Read the model definition and answer for the solid it produces. Units are mm, in the model's axes. Face numbers are marked on the shaded views. A direction names the side the tool comes from. Give positions to 0.01 mm unless a question says otherwise; leave off trailing zeros. Write each loop counter-clockwise with the first axis right and the second up, starting at its lowest first coordinate (ties: lowest second). Pieces come first, ordered by that corner, then holes. Notation, with made-up numbers: M 33,73 L 60,73 A16 ccw 60,77 Z; hole C 36.25,-25.75 d10. An arc over 180 degrees is marked long. Use a Markdown table: item, result. Add a question column.
Item 1: A cutting plane is placed at B-B on x = -33. Count the separate pieces of the cut face and the enclosed holes in it, then the cut area to 3 significant figures.
Item 2: A cutting plane is placed at A-A on z = 4.25. Determine the outline of the cut face in (x, y).
Item 3: Given P1, Ø13, axis at x = 0.01, y = -11.72, coming from the -Z side; P2, Ø4, axis at x = 51, y = 19.5, coming from the +Z side, each flat-ended and moving along its own axis, determine where each tip first touches the part or whether it passes through.
Item 4: A cutting plane is placed at C-C on x = -70. Determine the outline of the cut face in (y, z), then the cut area to 3 significant figures.
Item 5: For the marked faces 1 and 2, determine the directions among +Z, -Z, +X, -X, +Y, -Y from which every point of the face is accessible in a straight line to the end or side of a thin tool.
Item 6: Consider probe 1 along Y at (x, z) = (-70, 1.2); probe 2 along Y at (x, z) = (47, 5.75); probe 3 along Z at (x, y) = (-17, 66). Determine where each line is inside the solid, lowest interval first. Write a range as [from, to].
Item 7: A cutting plane is placed at D-D on y = 62.5. Determine the outline of the cut face in (x, z).
from build123d import *

# Parameters (mm, degrees)
SKETCH_W      = 150
SKETCH_H      = 150
SKETCH_R      = 4
SKETCH_R_2    = 2
PAD_DEPTH     = 3
SKETCH001_R   = 4
SKETCH001_R_2 = 2
PAD001_DEPTH  = 4


with BuildPart() as part:
    # Sketch → Pad (new body)
    with BuildSketch(Plane.XY):
        Rectangle(SKETCH_W, SKETCH_H)
        with Locations((-23.457463, 46.865997)):
            Circle(SKETCH_R, mode=Mode.SUBTRACT)
        with Locations((-11.738286, 46.871353)):
            Circle(SKETCH_R, mode=Mode.SUBTRACT)
        with Locations((-0.019109, 46.876709)):
            Circle(SKETCH_R, mode=Mode.SUBTRACT)
        with Locations((11.700068, 46.882065)):
            Circle(SKETCH_R, mode=Mode.SUBTRACT)
        with Locations((23.419245, 46.887421)):
            Circle(SKETCH_R, mode=Mode.SUBTRACT)
        with Locations((-35.173599, 35.141463)):
            Circle(SKETCH_R, mode=Mode.SUBTRACT)
        with Locations((-23.454422, 35.146819)):
            Circle(SKETCH_R, mode=Mode.SUBTRACT)
        with Locations((-11.735245, 35.152175)):
            Circle(SKETCH_R, mode=Mode.SUBTRACT)
        with Locations((-0.016068, 35.157531)):
            Circle(SKETCH_R, mode=Mode.SUBTRACT)
        with Locations((11.703109, 35.162887)):
            Circle(SKETCH_R, mode=Mode.SUBTRACT)
        with Locations((23.422286, 35.168243)):
            Circle(SKETCH_R, mode=Mode.SUBTRACT)
        with Locations((35.141463, 35.173599)):
            Circle(SKETCH_R, mode=Mode.SUBTRACT)
        with Locations((-46.88742, 23.41693)):
            Circle(SKETCH_R, mode=Mode.SUBTRACT)
        with Locations((-35.168243, 23.422286)):
            Circle(SKETCH_R, mode=Mode.SUBTRACT)
        with Locations((-23.449066, 23.427642)):
            Circle(SKETCH_R, mode=Mode.SUBTRACT)
        with Locations((-11.729889, 23.432998)):
            Circle(SKETCH_R, mode=Mode.SUBTRACT)
        with Locations((-0.010712, 23.438354)):
            Circle(SKETCH_R, mode=Mode.SUBTRACT)
        with Locations((11.708465, 23.44371)):
            Circle(SKETCH_R, mode=Mode.SUBTRACT)
        with Locations((23.427642, 23.449066)):
            Circle(SKETCH_R, mode=Mode.SUBTRACT)
        with Locations((35.146819, 23.454422)):
            Circle(SKETCH_R, mode=Mode.SUBTRACT)
        with Locations((46.865996, 23.459778)):
            Circle(SKETCH_R, mode=Mode.SUBTRACT)
        with Locations((-46.882064, 11.697753)):
            Circle(SKETCH_R, mode=Mode.SUBTRACT)
        with Locations((-35.162887, 11.703109)):
            Circle(SKETCH_R, mode=Mode.SUBTRACT)
        with Locations((-23.44371, 11.708465)):
            Circle(SKETCH_R, mode=Mode.SUBTRACT)
        with Locations((-11.724533, 11.713821)):
            Circle(SKETCH_R, mode=Mode.SUBTRACT)
        with Locations((-0.005356, 11.719177)):
            Circle(SKETCH_R, mode=Mode.SUBTRACT)
        with Locations((11.713821, 11.724533)):
            Circle(SKETCH_R, mode=Mode.SUBTRACT)
        with Locations((23.432998, 11.729889)):
            Circle(SKETCH_R, mode=Mode.SUBTRACT)
        with Locations((35.152175, 11.735245)):
            Circle(SKETCH_R, mode=Mode.SUBTRACT)
        with Locations((46.871352, 11.740601)):
            Circle(SKETCH_R, mode=Mode.SUBTRACT)
        with Locations((-46.876708, -0.021424)):
            Circle(SKETCH_R, mode=Mode.SUBTRACT)
        with Locations((-35.157531, -0.016068)):
            Circle(SKETCH_R, mode=Mode.SUBTRACT)
        with Locations((-23.438354, -0.010712)):
            Circle(SKETCH_R, mode=Mode.SUBTRACT)
        with Locations((-11.719177, -0.005356)):
            Circle(SKETCH_R, mode=Mode.SUBTRACT)
        Circle(SKETCH_R, mode=Mode.SUBTRACT)
        with Locations((11.719177, 0.005356)):
            Circle(SKETCH_R, mode=Mode.SUBTRACT)
        with Locations((23.438354, 0.010712)):
            Circle(SKETCH_R, mode=Mode.SUBTRACT)
        with Locations((35.157531, 0.016068)):
            Circle(SKETCH_R, mode=Mode.SUBTRACT)
        with Locations((46.876708, 0.021424)):
            Circle(SKETCH_R, mode=Mode.SUBTRACT)
        with Locations((-46.871352, -11.740601)):
            Circle(SKETCH_R, mode=Mode.SUBTRACT)
        with Locations((-35.152175, -11.735245)):
            Circle(SKETCH_R, mode=Mode.SUBTRACT)
        with Locations((-23.432998, -11.729889)):
            Circle(SKETCH_R, mode=Mode.SUBTRACT)
        with Locations((-11.713821, -11.724533)):
            Circle(SKETCH_R, mode=Mode.SUBTRACT)
        with Locations((0.005356, -11.719177)):
            Circle(SKETCH_R, mode=Mode.SUBTRACT)
        with Locations((11.724533, -11.713821)):
            Circle(SKETCH_R, mode=Mode.SUBTRACT)
        with Locations((23.44371, -11.708465)):
            Circle(SKETCH_R, mode=Mode.SUBTRACT)
        with Locations((35.162887, -11.703109)):
            Circle(SKETCH_R, mode=Mode.SUBTRACT)
        with Locations((46.882064, -11.697753)):
            Circle(SKETCH_R, mode=Mode.SUBTRACT)
        with Locations((-46.865996, -23.459778)):
            Circle(SKETCH_R, mode=Mode.SUBTRACT)
        with Locations((-35.146819, -23.454422)):
            Circle(SKETCH_R, mode=Mode.SUBTRACT)
        with Locations((-23.427642, -23.449066)):
            Circle(SKETCH_R, mode=Mode.SUBTRACT)
        with Locations((-11.708465, -23.44371)):
            Circle(SKETCH_R, mode=Mode.SUBTRACT)
        with Locations((0.010712, -23.438354)):
            Circle(SKETCH_R, mode=Mode.SUBTRACT)
        with Locations((11.729889, -23.432998)):
            Circle(SKETCH_R, mode=Mode.SUBTRACT)
        with Locations((23.449066, -23.427642)):
            Circle(SKETCH_R, mode=Mode.SUBTRACT)
        with Locations((35.168243, -23.422286)):
            Circle(SKETCH_R, mode=Mode.SUBTRACT)
        with Locations((46.88742, -23.41693)):
            Circle(SKETCH_R, mode=Mode.SUBTRACT)
        with Locations((-35.141463, -35.173599)):
            Circle(SKETCH_R, mode=Mode.SUBTRACT)
        with Locations((-23.422286, -35.168243)):
            Circle(SKETCH_R, mode=Mode.SUBTRACT)
        with Locations((-11.703109, -35.162887)):
            Circle(SKETCH_R, mode=Mode.SUBTRACT)
        with Locations((0.016068, -35.157531)):
            Circle(SKETCH_R, mode=Mode.SUBTRACT)
        with Locations((11.735245, -35.152175)):
            Circle(SKETCH_R, mode=Mode.SUBTRACT)
        with Locations((23.454422, -35.146819)):
            Circle(SKETCH_R, mode=Mode.SUBTRACT)
        with Locations((35.173599, -35.141463)):
            Circle(SKETCH_R, mode=Mode.SUBTRACT)
        with Locations((-23.416872, -46.88742)):
            Circle(SKETCH_R, mode=Mode.SUBTRACT)
        with Locations((-11.697695, -46.882064)):
            Circle(SKETCH_R, mode=Mode.SUBTRACT)
        with Locations((0.021482, -46.876708)):
            Circle(SKETCH_R, mode=Mode.SUBTRACT)
        with Locations((11.740659, -46.871352)):
            Circle(SKETCH_R, mode=Mode.SUBTRACT)
        with Locations((23.459836, -46.865996)):
            Circle(SKETCH_R, mode=Mode.SUBTRACT)
        with Locations((-47.999982, 47.941119)):
            Circle(SKETCH_R_2, mode=Mode.SUBTRACT)
        with Locations((48, 48)):
            Circle(SKETCH_R_2, mode=Mode.SUBTRACT)
        with Locations((-47.941101, -48.058863)):
            Circle(SKETCH_R_2, mode=Mode.SUBTRACT)
        with Locations((48.058881, -47.999982)):
            Circle(SKETCH_R_2, mode=Mode.SUBTRACT)
        with Locations((-70, 70)):
            Circle(SKETCH_R_2, mode=Mode.SUBTRACT)
        with Locations((69.999974, 69.915361)):
            Circle(SKETCH_R_2, mode=Mode.SUBTRACT)
        with Locations((-70.084639, -69.999974)):
            Circle(SKETCH_R_2, mode=Mode.SUBTRACT)
        with Locations((69.915335, -70.084614)):
            Circle(SKETCH_R_2, mode=Mode.SUBTRACT)
    extrude(amount=PAD_DEPTH)

    # Sketch001 (on DatumPlane) → Pad001 (join)
    with BuildSketch(Plane.XY.offset(3)):
        with Locations((-48.014584, 47.985412)):
            Circle(SKETCH001_R)
        with Locations((-48.014584, 47.985412)):
            Circle(SKETCH001_R_2, mode=Mode.SUBTRACT)
        with Locations((47.985412, 48.014584)):
            Circle(SKETCH001_R)
        with Locations((47.985412, 48.014584)):
            Circle(SKETCH001_R_2, mode=Mode.SUBTRACT)
        with Locations((-47.985412, -48.014584)):
            Circle(SKETCH001_R)
        with Locations((-47.985412, -48.014584)):
            Circle(SKETCH001_R_2, mode=Mode.SUBTRACT)
        with Locations((48.014584, -47.985412)):
            Circle(SKETCH001_R)
        with Locations((48.014584, -47.985412)):
            Circle(SKETCH001_R_2, mode=Mode.SUBTRACT)
    extrude(amount=PAD001_DEPTH)


solid = part.part
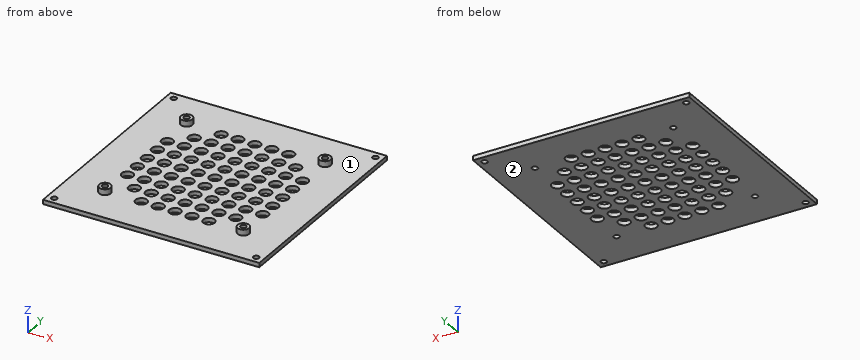
Filled in:
| question | item | result |
|---|---|---|
| 1 | separate pieces | 8 |
| 1 | enclosed holes | 0 |
| 1 | area | 309 mm² |
| 2 | outline | C -48.01,47.99 d8; C -47.99,-48.01 d8; C 47.99,48.01 d8; C 48.01,-47.99 d8; hole C -48.01,47.99 d4; hole C -47.99,-48.01 d4; hole C 47.99,48.01 d4; hole C 48.01,-47.99 d4 |
| 3 | P1 | z = 0 |
| 3 | P2 | z = 3 |
| 4 | outline | M -75,0 L -72,0 L -72,3 L -75,3 Z; M -68,0 L 68,0 L 68,3 L -68,3 Z; M 72,0 L 75,0 L 75,3 L 72,3 Z |
| 4 | area | 426 mm² |
| 5 | face 1 | +Z |
| 5 | face 2 | -Z, +X, -X, +Y, -Y |
| 6 | probe 1 | [-75, -72], [-68, 68], [72, 75] |
| 6 | probe 2 | [-51.85, -49.71], [-46.26, -44.12], [44.14, 46.27], [49.75, 51.89] |
| 6 | probe 3 | [0, 3] |
| 7 | outline | M -75,0 L 75,0 L 75,3 L -75,3 Z |
